Geometry: final body of the model. Coordinates: model frame, mm. A direction names the side the tool comes from. Round coordinates to 2 decimals unless told otherwise and drop trailing zeros. Loops run counter-clockwise (first coordinate to the right, second up) from the corner with the lowest first, then second, coordinate; pieces in that order, holes last. Notation, with made-up numbers: (-32, 1) - (7, 1) arc R15 cw to (7, 14) - close; hole circle Ø4 at (86, -15). An arc over 180 degrees is marked (long way). Return JSON: item names as keys, results as strings. Group by question number.
1. Section B-B on y = 16.75. Return loops of the section in (x, z), and give its area (3 significant figures).
2. First-contact query: pin 1 Ø3 at (x, y) = (3, 14.5) entering from +Z; pin 2 Ø1.4 at (x, z) = (1.5, 2.5) entering from -Y; pin 3 Ø6 at (y, z) = (2.5, -4) entering from +X. Flat tips, straight axial feed; report the tip coordinate or a pass-through.
3. Section C-C on x = 1. Return loops of the section in (y, z).
4. Material intervals for probe 1 along X at (y, z) = (18.5, 0); probe 2 along Y at (x, z) = (-2.05, 0); probe 3 along Y at (x, z) = (1.5, 3), sorted ascending.
5. Section D-D on y = 11.75. Return loops of the section in (x, z), and give its area (3 significant figures).
6. Set-up query: faces 4 (the face through (4.762, 18, 0)), 5 (the face through (3, 12.7, 0)). Return all of +Z, -Z, +X, -X, +Y, -Y with unobstructed straight access to the full face (end or side cutting, diameter ignored); none if empty.
7. Draft query along Z for faces 1 (the face through (-0.99, 9.26, -0.02)), 2 (the face through (0, 8, 3)), 3 (the face through (-2.47, 16.42, -0.32)). Return one class per face: +Z half, -Z half, draft (parallel to the pull), parting line (faces both ways), or undercut.
8. Section A-A on z = 0. Return loops of the section in (x, y), and give its area (3 significant figures).
Autodesk Inventor part; units mm, degrees
ref_plane "YZ Plane" through (0, 0, 0) normal (1, 0, 0) x (0, 1, 0)
ref_plane "XZ Plane" through (0, 0, 0) normal (0, 1, 0) x (-1, 0, 0)
ref_plane "XY Plane" through (0, 0, 0) normal (0, 0, 1) x (1, 0, 0)
sketch "Sketch1" plane through (0, 0, 0) normal (0, 1, 0) x (-1, 0, 0)
  line L0 (0, 0) -> (4.7625, 0)
  line L1 (4.7625, 0) -> (4.7625, -2.7496)
  line L2 (4.7625, 0) -> (7.5121, 0) construction
  line L3 (4.7625, 0) -> (4.7625, 2.7496)
  line L4 (2.3813, 4.1244) -> (0, 5.4993)
  line L5 (2.3813, 4.1244) -> (4.7625, 2.7496)
  line L6 (-2.3813, 4.1244) -> (-4.7625, 2.7496)
  line L7 (-2.3813, 4.1244) -> (0, 5.4993)
  line L8 (-4.7625, 0) -> (-4.7625, -2.7496)
  line L9 (-4.7625, 0) -> (-4.7625, 2.7496)
  line L10 (-2.3812, -4.1244) -> (0, -5.4993)
  line L11 (-2.3812, -4.1244) -> (-4.7625, -2.7496)
  line L12 (2.3813, -4.1244) -> (4.7625, -2.7496)
  line L13 (2.3813, -4.1244) -> (0, -5.4993)
  line L14 (4.7625, 2.7496) -> (4.7625, -2.7496)
  line L15 (4.7625, -2.7496) -> (0, -5.4993)
  line L16 (0, -5.4993) -> (-4.7625, -2.7496)
  line L17 (-4.7625, -2.7496) -> (-4.7625, 2.7496)
  line L18 (-4.7625, 2.7496) -> (0, 5.4993)
  line L19 (4.7625, 2.7496) -> (0, 5.4993)
  dimension "d0" = 4.7625
  dimension "d1" = 90
  dimension "d4" = 360
extrude "Extrusion1" add sketch "Sketch1" along normal blind 22.86
sketch "Sketch2" plane through (0, 22.86, 0) normal (0, 1, 0) x (1, 0, 0)
  point P0 (0, 0)
  point P1 (0, 0)
hole "Hole1" at (0, 22.86, 0) direction (0, -1, 0) diameter 4.9784 depth 12.7 tip angle 118
sketch "Sketch3" plane through (0, 0, 0) normal (0, -1, 0) x (1, 0, 0)
  line L0 (0, 0) -> (9.2843, 0)
  line L1 (9.2843, 0) -> (9.2843, -7.4131)
  line L2 (9.2843, -7.4131) -> (0, -7.4131)
  line L3 (0, -7.4131) -> (0, 0)
  line L4 (9.2843, 0) -> (9.2843, 7.4131)
  line L5 (9.2843, 7.4131) -> (0, 7.4131)
  line L6 (0, 7.4131) -> (0, 0)
extrude "Extrusion2" cut sketch "Sketch3" against normal blind 12.7
sketch "Sketch5" plane through (0, 0, 5.4993) normal (1, 0, 0) x (0, 0, -1)
  line L0 (10.9985, 0) -> (10.9985, 12.7)
  line L1 (0, 0) -> (0, 12.7)
  line L2 (5.4993, 0) -> (5.4993, 4.7625)
  circle A0 centre (5.4993, 4.7625) radius 3.3782
  dimension "d17" = 4.7625
  dimension "d18" = 6.7564
hole "Hole2" at (0, 4.7625, 0) direction (-1, 0, 0) diameter 6.7564 end through all
sketch "Sketch7" plane through (0, 0, 5.4993) normal (1, 0, 0) x (0, 0, -1)
  arc A0 (2.7496, 2.7999) -> (8.2489, 2.7999) centre (5.4993, 4.7625) ccw
  line L0 (10.9985, 0) -> (10.9985, 12.7)
  circle A1 centre (5.4993, 4.7625) radius 7.2748
  point P0 (5.4993, 0)
properties part number "feet type 3 part 1 hexagon stock"
Taken from the geometry:
{
 "1": {"outline": "(-4.76, -2.75) - (-2.38, -4.12) - (0, -5.5) - (2.38, -4.12) - (4.76, -2.75) - (4.76, 2.75) - (2.38, 4.12) - (0, 5.5) - (-2.38, 4.12) - (-4.76, 2.75) - close; hole circle Ø4.98 at (0, 0)", "area": "59.1 mm2"},
 "2": {"pin 1": "z = 4.63", "pin 2": "y = 12.7", "pin 3": "x = 0"},
 "3": {"outline": "(12.7, -4.92) - (22.86, -4.92) - (22.86, -2.28) - (12.7, -2.28) - close; (12.7, 2.28) - (22.86, 2.28) - (22.86, 4.92) - (12.7, 4.92) - close"},
 "4": {"probe 1": "-4.76 to -2.49, 2.49 to 4.76", "probe 2": "0 to 1.38, 8.14 to 9.9", "probe 3": "12.7 to 22.86"},
 "5": {"outline": "(-4.76, -2.75) - (-2.38, -4.12) - (0, -5.5) - (0, -2.49) arc R2.49 cw to (0, 2.49) - (0, 5.5) - (-2.38, 4.12) - (-4.76, 2.75) - close", "area": "29.6 mm2"},
 "6": {"face 4": "+Z, -Z, +X, +Y, -Y", "face 5": "+Z, -Z, +X, -Y"},
 "7": {"face 1": "undercut", "face 2": "draft", "face 3": "undercut"},
 "8": {"outline": "(-4.76, 0) - (0, 0) - (0, 1.38) - (-4.76, 1.38) - close; (-4.76, 8.14) - (0, 8.14) - (0, 8.66) - (-2.49, 10.16) - (-2.49, 22.86) - (-4.76, 22.86) - close; (2.49, 12.7) - (4.76, 12.7) - (4.76, 22.86) - (2.49, 22.86) - close", "area": "66.3 mm2"}
}
